Read the model definition and answer for the solid it produces. Units are mm, in the model's axes. Round coordinates to 2 decimals unless told otherwise and drop trailing zeros. Write each loop counter-clockwise with the first axis right and the second up, starting at its lowest first coordinate (ties: lowest second). Pieces come first, ordered by that corner, then holes. Notation, with made-up numbers: (-21, 81.5) - (-13, 81.5) arc R21 ccw to (-13, 110.5) - close; hole circle Ø8 at (45, 32.5). An arc over 180 degrees is marked (long way). Answer as CSV lines item,"result". Start each with the question number.
1) Find section A-A on x = 25.4. Determine the outline of the cut face in (y, z).
2) Find section B-B on y = 4. State how many separate pieces and enclosed holes the cut face has, then the cut area to 3 significant figures.
3) Consider line 1 along X through (y, z) = (6.25, -14.5); line 2 along Z through (x, y) = (25.4, 0.8); line 3 along Z through (x, y) = (37, 2.75). Determine where each line is inside the solid, lowest interval first.
4) Each of these flat-tipped pins is pushed along its axis until it touches: pin 1 (8 mm diameter, centred on x = 15.875, z = -9.525, fed in from +Y); pin 2 (1 mm diameter, centred on y = 2, z = -20, fed in from -X); pin 3 (4 mm diameter, centred on x = 34.925, z = -9.525, fed in from -Y). Where does it stop, or does it pass through?
from build123d import *

# Parameters (mm, degrees)
SKETCH1_W                                     = 50.8
SKETCH1_H                                     = 95.25
BOSS_EXTRUDE1_DEPTH                           = 6.35
CSK_FOR_1_4_FLAT_HEAD_MACHINE_SCREW1_AT_COUNT = 2
CSK_FOR_1_4_FLAT_HEAD_MACHINE_SCREW1_AT_PITCH = 59.504785784
CSK_FOR_1_4_FLAT_HEAD_MACHINE_SCREW1_2_COUNT  = 2
CSK_FOR_1_4_FLAT_HEAD_MACHINE_SCREW1_2_PITCH  = 59.504785784


with BuildPart() as part:
    # Sketch1 → Boss-Extrude1 (new body)
    with BuildSketch(Plane(origin=(0, 0, 0), x_dir=(1, 0, 0), z_dir=(0, 1, 0))):
        with Locations((25.4, 47.625)):
            Rectangle(SKETCH1_W, SKETCH1_H)
    extrude(amount=BOSS_EXTRUDE1_DEPTH)

    # Sketch4 → CSK for 1/4 Flat Head Machine Screw1 (revolve, cut)
    with BuildSketch(Plane(origin=(25.4, 6.35, -68.2625), x_dir=(0, 0, 1), z_dir=(1, 0, 0))):
        Polygon((0, 0), (0, 6.35), (3.3782, 6.35), (3.3782, 3.520932584), (6.4389, 0), align=None)
    csk_for_1_4_flat_head_machine_screw1 = revolve(axis=Axis((25.4, 12.7, -68.2625), (0, -1, 0)), mode=Mode.SUBTRACT)

    # CSK for 1/4 Flat Head Machine Screw1 at: CSK for 1/4 Flat Head Machine Screw1 ×2
    with Locations(*[Vector(-0.16007115855366244, 0, 0.9871054777475852) * (i * CSK_FOR_1_4_FLAT_HEAD_MACHINE_SCREW1_AT_PITCH) for i in range(1, CSK_FOR_1_4_FLAT_HEAD_MACHINE_SCREW1_AT_COUNT)]):
        add(csk_for_1_4_flat_head_machine_screw1, mode=Mode.SUBTRACT)

    # CSK for 1_4 Flat Head Machine Screw1 2: CSK for 1/4 Flat Head Machine Screw1 ×2
    with Locations(*[Vector(0.16007115855366244, 0, 0.9871054777475852) * (i * CSK_FOR_1_4_FLAT_HEAD_MACHINE_SCREW1_2_PITCH) for i in range(1, CSK_FOR_1_4_FLAT_HEAD_MACHINE_SCREW1_2_COUNT)]):
        add(csk_for_1_4_flat_head_machine_screw1, mode=Mode.SUBTRACT)


solid = part.part
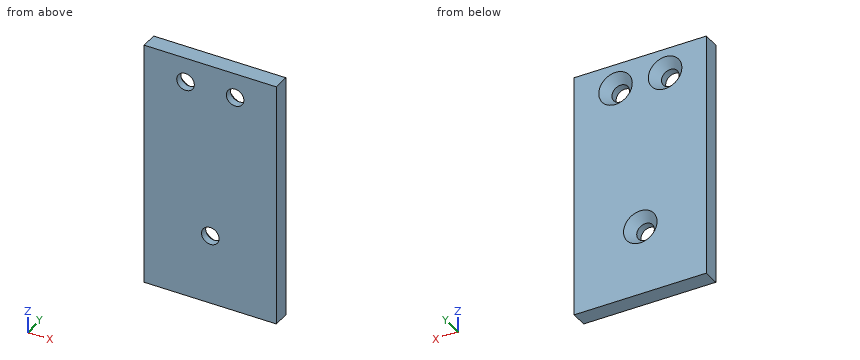
Check values:
1,outline,"(0, -95.25) - (6.35, -95.25) - (6.35, -74.7) - (2.83, -71.64) - (0, -71.64) - close; (0, -64.88) - (2.83, -64.88) - (6.35, -61.82) - (6.35, 0) - (0, 0) - close"
2,separate pieces,"1"
2,enclosed holes,"3"
2,area,"4,660 mm^2"
3,line 1,"x = 0 to 11.93, 19.82 to 30.98, 38.87 to 50.8"
3,line 2,"z = -95.25 to -71.64, -64.88 to 0"
3,line 3,"z = -95.25 to -12.19, -6.86 to 0"
4,pin 1,"stops at y = 3.54"
4,pin 2,"stops at x = 0"
4,pin 3,"passes through"
